Design review of the part built by this model. Coordinates are the model's own, in mm. A direction names the side the tool comes from. Give positions to 0.01 mm unless a question says otherwise; leave off trailing zeros. Order: outer loops, then holes, each group sorted by start corner. A loop starts at its lowest first (then second) coordinate and runs counter-clockwise, first axis right, second up. Notation, with made-up numbers: (37, 43) - (65, 43) arc R24 ccw to (65, 74) - close; hole circle Ø2 at (46, 23). An arc over 180 degrees is marked (long way). Write each question's results on one line, items separated by ' | '. Start each with the question number.
```python
from build123d import *

# Parameters (mm, degrees)
SKETCH1_R           = 40
SKETCH1_R_2         = 20
BOSS_EXTRUDE1_DEPTH = 110
SKETCH2_R           = 50
SKETCH2_R_2         = 20
BOSS_EXTRUDE2_DEPTH = 10
SKETCH3_W           = 12
SKETCH3_H           = 14.623455079
CUT_EXTRUDE1_DEPTH  = 131.766968306


with BuildPart() as part:
    # Sketch1 → Boss-Extrude1 (new body)
    with BuildSketch(Plane.XY):
        Circle(SKETCH1_R)
        Circle(SKETCH1_R_2, mode=Mode.SUBTRACT)
    extrude(amount=BOSS_EXTRUDE1_DEPTH)

    # Sketch2 → Boss-Extrude2 (add)
    with BuildSketch(Plane.XY.offset(25)):
        Circle(SKETCH2_R)
        Circle(SKETCH2_R_2, mode=Mode.SUBTRACT)
    extrude(amount=BOSS_EXTRUDE2_DEPTH)

    # Sketch3 → Cut-Extrude1 (cut, through all)
    with BuildSketch(Plane(origin=(0, 0, 0), x_dir=(-1, 0, 0), z_dir=(0, 0, -1))):
        with Locations((0, 17.688272461)):
            Rectangle(SKETCH3_W, SKETCH3_H)
    extrude(amount=-CUT_EXTRUDE1_DEPTH, mode=Mode.SUBTRACT)


solid = part.part
```
Q1. Add section C-C (z = 62). Give the boundary of the cut face in (x, y), plus the area to 3 significant figures.
Q2. For line 1 (Y direction, x = 0, z = 23); line 2 (X direction, y = 0, z = 77); line 3 (Z direction, x = -36, y = -34.5), list the stretches that pass through material, from the lowest coordinate up. Write a range as [from, to].
Q3. Insertion check: pin 1 Ø9.5 at (x, z) = (0, 65.5) entering from -Y; pin 2 Ø24 at (x, y) = (0, 0) entering from +Z; pin 3 Ø3 at (y, z) = (21.5, 41) entering from -X; pin 4 Ø5 at (y, z) = (23.5, 62.5) entering from +X. Each pin has a flat end and moves straight along its axis. Give the tip position at first contact, or say it passes through.
Q4. Add section B-B (x = 0). Give the boundary of the cut face in (y, z), plus the area to 3 significant figures.
Q5. Add section A-A (y = 0). Give the boundary of the cut face in (x, z).
Q6. Machinability: for faces 5 (the flat face through (-22, 34, 25)), 6 (the flat face through (-9.4, 18.3, 0)), 7 (the flat face through (0, 25, 54)), 8 (the cylindrical face through (-8.67, -39.05, 71.97)), which of the approach directions +Z, -Z, +X, -X, +Y, -Y give a long, thin tool a straight path to every point of the face, cutting with its end or side? Answer none if there is none.
Q7. Add section D-D (y = -37.5). Give the boundary of the cut face in (x, z), plus the area to 3 significant figures.
Q8. Draft analysis for pull direction X (two halves, no side actions). For faces 1 (the cylindrical face through (-0.794, -19.984, 54.23)), 2 (the flat face through (-9.4, 18.3, 110)), 3 (the cylindrical face through (-8.67, -39.05, 12.32)), 4 (the flat face through (6, 22, 54)), state which applies: pulls with the +X half, pulls with the -X half, needs draft (parallel to the pull), parting line crosses it, or undercut.
Verdict:
1) outline: circle Ø80 at (0, 0); hole (-6, 19.08) arc R20 ccw (long way) to (6, 19.08) - (6, 25) - (-6, 25) - close | area: 3,710 mm2
2) line 1: y = [-40, -20], [25, 40] | line 2: x = [-40, -20], [20, 40] | line 3: z = [25, 35]
3) pin 1: stops at y = -40 | pin 2: passes through | pin 3: stops at x = -34.64 | pin 4: stops at x = 34.04
4) outline: (-50, 25) - (-40, 25) - (-40, 0) - (-20, 0) - (-20, 110) - (-40, 110) - (-40, 35) - (-50, 35) - close; (25, 0) - (40, 0) - (40, 25) - (50, 25) - (50, 35) - (40, 35) - (40, 110) - (25, 110) - close | area: 4,050 mm2
5) outline: (-50, 25) - (-40, 25) - (-40, 0) - (-20, 0) - (-20, 110) - (-40, 110) - (-40, 35) - (-50, 35) - close; (20, 0) - (40, 0) - (40, 25) - (50, 25) - (50, 35) - (40, 35) - (40, 110) - (20, 110) - close
6) face 5: -Z | face 6: -Z, +X, -X, +Y, -Y | face 7: +Z, -Z | face 8: +Z
7) outline: (-33.07, 25) - (-13.92, 25) - (-13.92, 0) - (13.92, 0) - (13.92, 25) - (33.07, 25) - (33.07, 35) - (13.92, 35) - (13.92, 110) - (-13.92, 110) - (-13.92, 35) - (-33.07, 35) - close | area: 3,450 mm2
8) face 1: undercut | face 2: needs draft | face 3: parting line crosses it | face 4: undercut
